```python
from build123d import *

# Parameters (mm, degrees)
ESQUISSE1_W             = 106
ESQUISSE1_H             = 136
BOSS_EXTRU_1_DEPTH      = 3
CONG_1_R                = 3
ESQUISSE2_R             = 6
ENL_V_MAT_EXTRU_1_DEPTH = 10


with BuildPart() as part:
    # Esquisse1 → Boss.-Extru.1 (new body)
    with BuildSketch(Plane(origin=(0, 0, 0), x_dir=(1, 0, 0), z_dir=(0, 1, 0))):
        Rectangle(ESQUISSE1_W, ESQUISSE1_H)
    extrude(amount=BOSS_EXTRU_1_DEPTH)

    # Congé1
    cong_1_edges = [part.edges().sort_by_distance(p)[0] for p in [
        (53, 1.5, 68),
        (-53, 1.5, 68),
        (-53, 1.5, -68),
        (53, 1.5, -68),
    ]]
    fillet(cong_1_edges, radius=CONG_1_R)

    # Esquisse2 → Enlèv. mat.-Extru.1 (cut)
    with BuildSketch(Plane(origin=(0, 3, 0), x_dir=(1, 0, 0), z_dir=(0, 1, 0))):
        with Locations((-35, -58.6)):
            Circle(ESQUISSE2_R)
        with Locations((-10, -38)):
            Circle(ESQUISSE2_R)
    extrude(amount=-ENL_V_MAT_EXTRU_1_DEPTH, mode=Mode.SUBTRACT)


solid = part.part
```
Geometry: final body of the model. Coordinates: model frame, mm. Coordinates: 2 decimals unless noted, no trailing zeros. Order: outer loops, then holes, each group sorted by start corner. A loop starts at its lowest first (then second) coordinate and runs counter-clockwise, first axis right, second up. Notation, with made-up numbers: M -33.75,17.25 L -26.75,17.25 A27 ccw -26.75,48.25 Z; hole C 62.25,25.5 d8. An arc over 180 degrees is marked long. Answer in a Markdown table with one row per item. Add a question column.
Q1. Mould query, pull axis Z, two halves, no side actions, for faces 1 (the cylindrical face through (-11.301, 1.521, 43.857)), 2 (the flat face through (53, 1, 1)), 3 (the flat face through (-1, 1, 68)), 4 (the cylindrical face through (-52.14, 1.52, -67.1)). Classes: released by +Z, released by -Z, zero draft, split by the parting line, or undercut.
Q2. Line query: L1, parallel to X at y = 2, z = 58.6; L2, parallel to X at y = 1.4, z = 38; L3, parallel to Z at x = -10, y = 0.8. Output: solid intervals per line, ascending.
Q3. Section query A-A on x = -10. Return the cut outline in (y, z), and give its area (3 significant figures).
Q4. Section query C-C on y = 0.5. Return the cut outline in (x, z).
Q5. Section query B-B on z = 58.6. Return the cut outline in (x, y).
Completed:
| question | item | result |
|---|---|---|
| 1 | face 1 | undercut |
| 1 | face 2 | zero draft |
| 1 | face 3 | released by +Z |
| 1 | face 4 | released by -Z |
| 2 | L1 | x = -53 to -41, -29 to 53 |
| 2 | L2 | x = -53 to -16, -4 to 53 |
| 2 | L3 | z = -68 to 32, 44 to 68 |
| 3 | outline | M 0,-68 L 3,-68 L 3,32 L 0,32 Z; M 0,44 L 3,44 L 3,68 L 0,68 Z |
| 3 | area | 372 mm2 |
| 4 | outline | M -53,-65 A3 ccw -50,-68 L 50,-68 A3 ccw 53,-65 L 53,65 A3 ccw 50,68 L -50,68 A3 ccw -53,65 Z; hole C -35,58.6 d12; hole C -10,38 d12 |
| 5 | outline | M -53,0 L -41,0 L -41,3 L -53,3 Z; M -29,0 L 53,0 L 53,3 L -29,3 Z |
